Design review of the part shown in the three views and the two pictorial views. Dimensions are in mm from the part's minimum x, y and z. Round coordinates to 2 decimals unless told otherwise and drop trailing zeros. Order: outer loops, then holes, each group sorted by start corner. A loop starts at its lowest first (then second) coordinate and runs counter-clockwise, first axis right, second up. Notation, with made-up numbers: (-20, 82.5) - (-12, 82.5) arc R11 cw to (-12, 87.5) - close; hole circle Ø7 at (7, 84.5). An arc over 180 degrees is marked (long way). One line per item, written item: value.
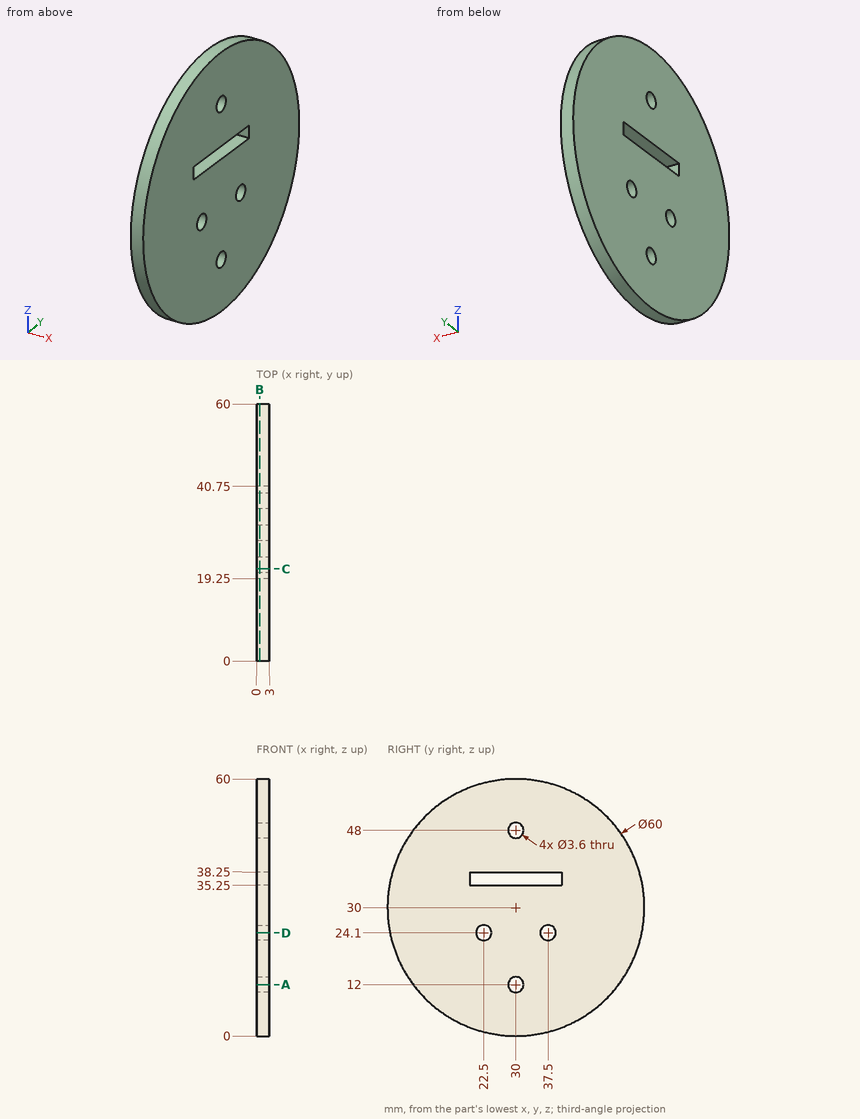
Item 1: Take a section at A-A (z = 12). Write out the cut boundary in (x, y), plus the area to 3 significant figures.
Returned:
outline: (0, 6) - (3, 6) - (3, 28.2) - (0, 28.2) - close; (0, 31.8) - (3, 31.8) - (3, 54) - (0, 54) - close
area: 133 mm^2
Item 2: For P1, Ø3, axis at y = 30, z = 12, coming from the +X side (3 decimals); P2, Ø1, axis at x = 1.5, z = 37.5, coming from the -Y side, all flat-tipped, find the tip position at first contact; note any pin that passes through.
Returned:
P1: through
P2: y = 0.83
Item 3: Wall thickness on line 1 (Y direction, x = 1, z = 24.1); line 2 (Y direction, x = 1.15, z = 36); line 3 (Y direction, x = 1.9, z = 11): over which ranges is each line inside the solid? List them lowest first.
Returned:
line 1: 0.59 to 20.7, 24.3 to 35.7, 39.3 to 59.41
line 2: 0.61 to 19.25, 40.75 to 59.39
line 3: 6.78 to 28.5, 31.5 to 53.22
Item 4: Take a section at D-D (z = 24.1). Write out the cut boundary in (x, y), plus the area to 3 significant figures.
Returned:
outline: (0, 0.59) - (3, 0.59) - (3, 20.7) - (0, 20.7) - close; (0, 24.3) - (3, 24.3) - (3, 35.7) - (0, 35.7) - close; (0, 39.3) - (3, 39.3) - (3, 59.41) - (0, 59.41) - close
area: 155 mm^2
Item 5: Take a section at C-C (y = 21.5). Write out the cut boundary in (x, z).
Returned:
outline: (0, 1.23) - (3, 1.23) - (3, 22.6) - (0, 22.6) - close; (0, 25.6) - (3, 25.6) - (3, 35.25) - (0, 35.25) - close; (0, 38.25) - (3, 38.25) - (3, 58.77) - (0, 58.77) - close
Item 6: Take a section at B-B (x = 0.7). Write out the cut boundary in (y, z).
Returned:
outline: circle Ø60 at (30, 30); hole (19.25, 35.25) - (40.75, 35.25) - (40.75, 38.25) - (19.25, 38.25) - close; hole circle Ø3.6 at (22.5, 24.1); hole circle Ø3.6 at (30, 12); hole circle Ø3.6 at (30, 48); hole circle Ø3.6 at (37.5, 24.1)
